CAD build for the part. Positions are in the model's coordinates, mm. Face numbers are marked on the shaded views. A direction names the side the tool comes from. Give positions to 0.01 mm unless a question says otherwise; leave off trailing zeros. Order: outer loops, then holes, each group sorted by start corner. A loop starts at its lowest first (then second) coordinate and runs counter-clockwise, first axis right, second up.
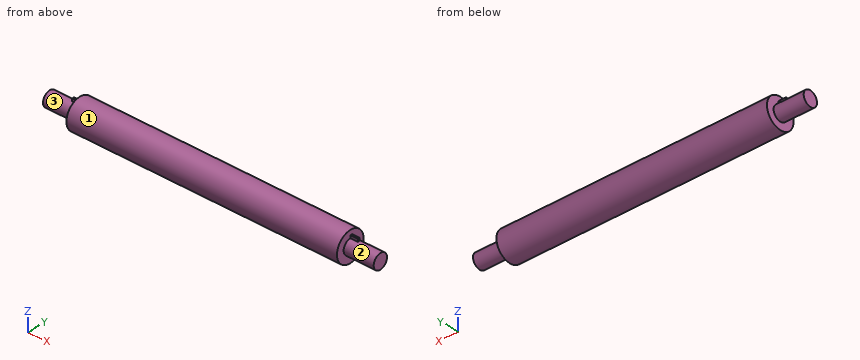
from build123d import *

# Parameters (mm, degrees)
BOSS_EXTRUDE1_DEPTH = 5


with BuildPart() as part:
    # Sketch1 → Revolve1 (revolve)
    with BuildSketch(Plane(origin=(0, 0, 0), x_dir=(1, 0, 0), z_dir=(0, 1, 0))):
        Polygon((-110, 0), (110, 0), (110, -5), (90, -5), (90, -10), (-90, -10), (-90, -5), (-110, -5), align=None)
    revolve(axis=Axis((-110, 0, 0), (1, 0, 0)))

    # Sketch2 → Boss-Extrude1 (add)
    with BuildSketch(Plane(origin=(90, 0, 0), x_dir=(0, 0, -1), z_dir=(1, 0, 0))):
        with BuildLine():
            Line((-5, 0), (-6.809348939, 0))
            Line((-6.809348939, 0), (-6.809348939, 1.307755756))
            Line((-6.809348939, 1.307755756), (-4.825948081, 1.307755756))
            ThreePointArc((-4.825948081, 1.307755756), (-4.956296016, 0.65964369), (-5, 0))
        make_face()
    boss_extrude1 = extrude(amount=BOSS_EXTRUDE1_DEPTH)

    # Mirror1: Boss-Extrude1 across plane
    add(boss_extrude1.mirror(Plane(origin=(0, 0, 0), x_dir=(0, 0, 1), z_dir=(1, 0, 0))))


solid = part.part
1. Saw through at B-B on y = 8. Give the cut face in (x, z), plus the area to 3 significant figures.
2. Saw through at C-C on x = 84. Give the cut face in (y, z), plus the area to 3 significant figures.
3. Wall check: line 1 (Z direction, x = 40.5, y = 0.5); line 2 (X direction, y = 5, z = 1.25); line 3 (Y direction, x = 82.5, z = 8.5). Give the ranges that are in metal, low to high.
4. 3-axis set-ups, long thin cutter, end or side, ignore diameter. For the marked faces 1, 2 and 3: which of +Z, -Z, +X, -X, +Y, -Y reach the whole face in a straight line?
5. Pin check, flat tips, straight feed: P1, Ø0.9, axis at x = -93, z = 6, coming from the -Y side; P2, Ø3, axis at x = 45.5, z = 7, coming from the +Y side; P3, Ø0.6, axis at x = -91.5, z = 5.5, coming from the +Y side. Stop position of each tip, or through.
6. Saw through at A-A on z = 0. Give the cut face in (x, y).
Reported:
1. outline: (-90, -6) - (90, -6) - (90, 6) - (-90, 6) - close
1. area: 2,160 mm2
2. outline: circle Ø20 at (0, 0)
2. area: 314 mm2
3. line 1: z = -9.99 to 9.99
3. line 2: x = -90 to 90
3. line 3: y = -5.27 to 5.27
4. face 1: +X, -X
4. face 2: +X
4. face 3: -X
5. P1: stops at y = 0
5. P2: stops at y = 8.35
5. P3: stops at y = 1.31
6. outline: (-110, -5) - (-90, -5) - (-90, -10) - (90, -10) - (90, -5) - (110, -5) - (110, 5) - (90, 5) - (90, 10) - (-90, 10) - (-90, 5) - (-110, 5) - close
